Geometry check sheet. Reference: the model listing, model coordinates, mm. A direction names the side the tool comes from. Give positions to 0.01 mm unless a question says otherwise; leave off trailing zeros. Write each loop counter-clockwise with the first axis right and the second up, starting at its lowest first coordinate (ties: lowest second). Pieces come first, ordered by that corner, then holes. Notation, with made-up numbers: (60, -32.75) - (112, -32.75) arc R36 cw to (112, 2.25) - close; hole circle Ø9 at (52, -4). An arc over 180 degrees is marked (long way). Write item = value, one per line. Start each with the question number.
(1) Depth check by flat-ended pin: pin 1 Ø4 at (x, y) = (-15, -438.5) entering from +Z; pin 2 Ø1 at (y, z) = (175.5, -6) entering from +X. Enter the tip coordinate at first touch or a pass-through.
(2) Thickness scan on L1, parallel to X at y = 546.1, z = -20; L2, parallel to X at y = -207.5, z = 1. Record the ranges inside material, lowest first.
(3) Section check A-A, the plane y = 352.5. Enter the section's corners in (x, z), plus the area to 3 significant figures.
(4) Access from +Z, -Z, +X, -X, +Y, -Y to the whole of each face (thin tool, end or side, straight path). Record for faces 1 (the flat face through (-20, -571.5, -7)), 2 (the flat face through (-18.263, -8, 3)).
(5) Section check B-B, the plane z = 12. Enter the section's corners in (x, y).
```python
from build123d import *

# Parameters (mm, degrees)
F1_DEPTH = 571.5
F3_D     = 8.89


with BuildPart() as f1:
    # F0 (on Front) → F1 (new body, symmetric)
    with BuildSketch(Plane.XZ):
        Polygon((-24.6126, -24.6126), (24.6126, -24.6126), (24.6126, -18.2626), (-18.2626, -18.2626), (-18.2626, 24.6126), (-24.6126, 24.6126), align=None)
    extrude(amount=F1_DEPTH, both=True)

    # F3 (through all)
    with Locations(Plane.XY.offset(-18.2626)):
        with Locations((-1.6002, -546.1), (-1.6002, 546.1)):
            Hole(F3_D / 2)


solid = f1.part
```
Model answer:
q1.pin_1 = -18.26
q1.pin_2 = -18.26
q2.L1 = -24.61 to -6.05, 2.84 to 24.61
q2.L2 = -24.61 to -18.26
q3.outline = (-24.61, -24.61) - (24.61, -24.61) - (24.61, -18.26) - (-18.26, -18.26) - (-18.26, 24.61) - (-24.61, 24.61) - close
q3.area = 585 mm²
q4.face_1 = +Z, -Z, +X, -X, -Y
q4.face_2 = +Z, +X, +Y, -Y
q5.outline = (-24.61, -571.5) - (-18.26, -571.5) - (-18.26, 571.5) - (-24.61, 571.5) - close
